The drawing under review shows one solid part. Ordinate dimensions are in mm from its lowest x, y, z. Give positions to 0.01 mm unless a question says otherwise; leave off trailing zeros. Loops run counter-clockwise (first coordinate to the right, second up) from the corner with the lowest first, then second, coordinate; pieces in that order, holes last. Notation, with made-up numbers: (-24.75, 69) - (-1.75, 69) arc R34 cw to (-1.75, 107) - close; hole circle Ø8 at (19.25, -11). An arc over 180 degrees is marked (long way). Return JSON: item names as keys, results as strings. Group by question number.
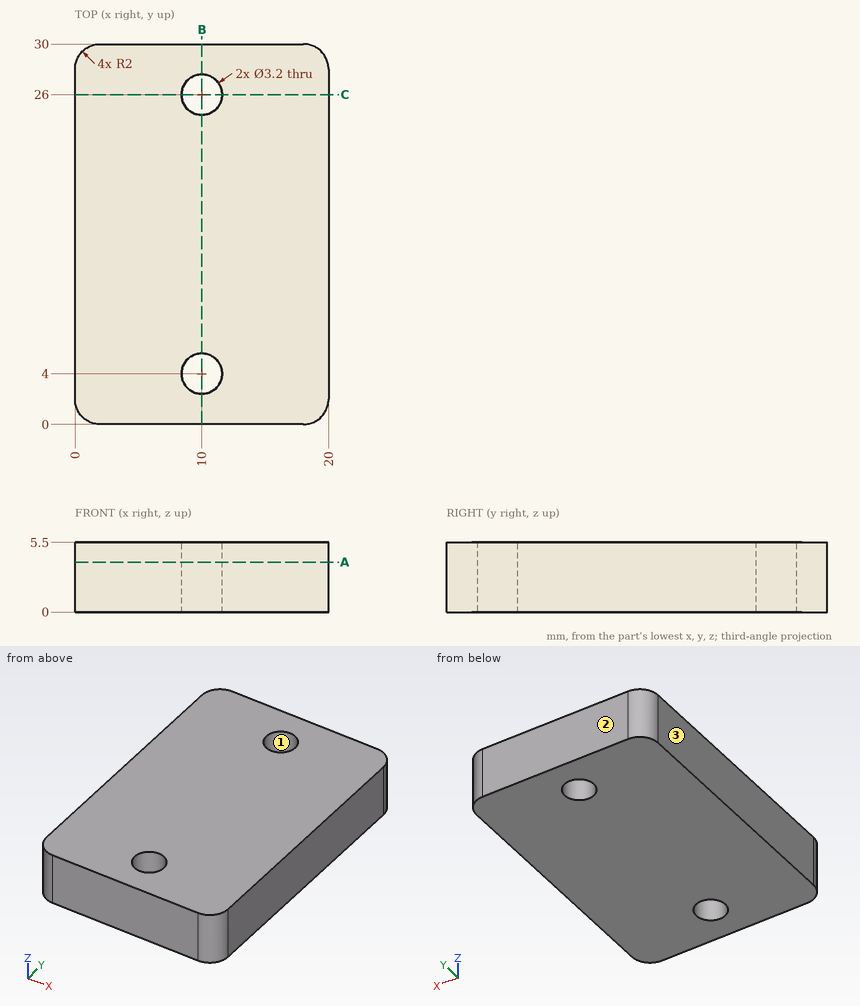
1) We need section A-A, the plane z = 3.95. Write out the cut boundary in (x, y).
2) We need section B-B, the plane x = 10. Write out the cut boundary in (y, z), plus the area to 3 significant figures.
3) Draft analysis for pull direction Y (two halves, no side actions). For the marked faces 1, 2 and 3, state which applies: +Y half, -Y half, draft (parallel to the pull), parting line (faces both ways), or undercut.
4) We need section C-C, the plane y = 26. Write out the cut boundary in (x, z), plus the area to 3 significant figures.
5) To check wall thickness, follow line 1 (Y direction, x = 10, z = 1.6); line 2 (X direction, y = 4, z = 2.3); line 3 (Y direction, x = 1.5, z = 4.8). State the ranges of each line that lie inside material, in increasing order.
Findings:
{
 "1": {"outline": "(0, 2) arc R2 ccw to (2, 0) - (18, 0) arc R2 ccw to (20, 2) - (20, 28) arc R2 ccw to (18, 30) - (2, 30) arc R2 ccw to (0, 28) - close; hole circle Ø3.2 at (10, 4); hole circle Ø3.2 at (10, 26)"},
 "2": {"outline": "(0, 0) - (2.4, 0) - (2.4, 5.5) - (0, 5.5) - close; (5.6, 0) - (24.4, 0) - (24.4, 5.5) - (5.6, 5.5) - close; (27.6, 0) - (30, 0) - (30, 5.5) - (27.6, 5.5) - close", "area": "130 mm^2"},
 "3": {"face 1": "undercut", "face 2": "+Y half", "face 3": "draft"},
 "4": {"outline": "(0, 0) - (8.4, 0) - (8.4, 5.5) - (0, 5.5) - close; (11.6, 0) - (20, 0) - (20, 5.5) - (11.6, 5.5) - close", "area": "92.4 mm^2"},
 "5": {"line 1": "y = 0 to 2.4, 5.6 to 24.4, 27.6 to 30", "line 2": "x = 0 to 8.4, 11.6 to 20", "line 3": "y = 0.06 to 29.94"}
}
